The model under review builds one solid part; all positions refer to its coordinate system, in mm. A direction names the side the tool comes from. Give positions to 0.01 mm unless a question says otherwise; leave off trailing zeros. Order: outer loops, then holes, each group sorted by start corner. A loop starts at its lowest first (then second) coordinate and runs counter-clockwise, first axis right, second up.
```python
from build123d import *

# Parameters (mm, degrees)
SKETCH1_W           = 10
SKETCH1_H           = 4
BOSS_EXTRUDE1_DEPTH = 1
SKETCH1_3_W         = 38
SKETCH1_3_H         = 1
BOSS_EXTRUDE2_DEPTH = 4
BOSS_EXTRUDE3_DEPTH = 23
SKETCH2_W           = 5
SKETCH2_H           = 3
BOSS_EXTRUDE4_DEPTH = 3
CUT_EXTRUDE1_DEPTH  = 56.873182297
BOSS_EXTRUDE5_DEPTH = 7
BOSS_EXTRUDE8_DEPTH = 23
SKETCH6_W           = 5
SKETCH6_H           = 3
BOSS_EXTRUDE9_DEPTH = 3
CUT_EXTRUDE3_DEPTH  = 56.873182297


with BuildPart() as part:
    # Sketch1 → Boss-Extrude1 (new body)
    with BuildSketch(Plane(origin=(0, 0, 0), x_dir=(1, 0, 0), z_dir=(0, 1, 0))):
        with BuildLine():
            Line((8.75, 22.5), (8.75, 12))
            ThreePointArc((8.75, 12), (8.530330086, 11.469669914), (8, 11.25))
            Line((8, 11.25), (0.75, 11.25))
            ThreePointArc((0.75, 11.25), (0.219669914, 11.469669914), (0, 12))
            Line((0, 12), (0, 1))
            ThreePointArc((0, 1), (0.292893219, 0.292893219), (1, 0))
            Line((1, 0), (43, 0))
            ThreePointArc((43, 0), (43.707106781, 0.292893219), (44, 1))
            Line((44, 1), (44, 33.5))
            ThreePointArc((44, 33.5), (43.707106781, 34.207106781), (43, 34.5))
            Line((43, 34.5), (1, 34.5))
            ThreePointArc((1, 34.5), (0.292893219, 34.207106781), (0, 33.5))
            Line((0, 33.5), (0, 22.5))
            ThreePointArc((0, 22.5), (0.219669914, 23.030330086), (0.75, 23.25))
            Line((0.75, 23.25), (8, 23.25))
            ThreePointArc((8, 23.25), (8.530330086, 23.030330086), (8.75, 22.5))
        make_face()
        with Locations((33.2, 26.7)):
            Rectangle(SKETCH1_W, SKETCH1_H, mode=Mode.SUBTRACT)
    extrude(amount=BOSS_EXTRUDE1_DEPTH)

    # Sketch1<3> → Boss-Extrude2 (add)
    # profile 1 of 12: a face of its own
    with BuildSketch(Plane(origin=(0, 0, 0), x_dir=(1, 0, 0), z_dir=(0, 1, 0))):
        with BuildLine():
            ThreePointArc((43.5, 35.5), (44.560660172, 35.060660172), (45, 34))
            Line((45, 34), (45, 0.5))
            ThreePointArc((45, 0.5), (44.560660172, -0.560660172), (43.5, -1))
            Line((43.5, -1), (0.5, -1))
            ThreePointArc((0.5, -1), (-0.560660172, -0.560660172), (-1, 0.5))
            Line((-1, 0.5), (-1, 34))
            ThreePointArc((-1, 34), (-0.560660172, 35.060660172), (0.5, 35.5))
            Line((0.5, 35.5), (43.5, 35.5))
        make_face()
        with BuildLine():
            ThreePointArc((1, 34.5), (0.292893219, 34.207106781), (0, 33.5))
            Line((0, 33.5), (0, 24.75))
            Line((0, 24.75), (0, 22.5))
            Line((0, 22.5), (0, 12))
            Line((0, 12), (0, 9.75))
            Line((0, 9.75), (0, 1))
            ThreePointArc((0, 1), (0.292893219, 0.292893219), (1, 0))
            Line((1, 0), (43, 0))
            ThreePointArc((43, 0), (43.707106781, 0.292893219), (44, 1))
            Line((44, 1), (44, 33.5))
            ThreePointArc((44, 33.5), (43.707106781, 34.207106781), (43, 34.5))
            Line((43, 34.5), (1, 34.5))
        make_face(mode=Mode.SUBTRACT)
    # profile 2 of 12: a face of its own
    with BuildSketch(Plane(origin=(0, 0, 0), x_dir=(1, 0, 0), z_dir=(0, 1, 0))):
        with BuildLine():
            Line((3, 0), (1, 0))
            ThreePointArc((1, 0), (0.292893219, 0.292893219), (0, 1))
            Line((0, 1), (0, 3))
            Line((0, 3), (-1, 3))
            Line((-1, 3), (-1, 0.5))
            ThreePointArc((-1, 0.5), (-0.560660172, -0.560660172), (0.5, -1))
            Line((0.5, -1), (3, -1))
            Line((3, -1), (3, 0))
        make_face()
    # profile 3 of 12: a face of its own
    with BuildSketch(Plane(origin=(0, 0, 0), x_dir=(1, 0, 0), z_dir=(0, 1, 0))):
        with Locations((22, -0.5)):
            Rectangle(SKETCH1_3_W, SKETCH1_3_H)
    # profile 4 of 12: a face of its own
    with BuildSketch(Plane(origin=(0, 0, 0), x_dir=(1, 0, 0), z_dir=(0, 1, 0))):
        with BuildLine():
            Line((43, 0), (41, 0))
            Line((41, 0), (41, -1))
            Line((41, -1), (43.5, -1))
            ThreePointArc((43.5, -1), (44.560660172, -0.560660172), (45, 0.5))
            Line((45, 0.5), (45, 3))
            Line((45, 3), (44, 3))
            Line((44, 3), (44, 1))
            ThreePointArc((44, 1), (43.707106781, 0.292893219), (43, 0))
        make_face()
    # profile 5 of 12: a face of its own
    with BuildSketch(Plane(origin=(0, 0, 0), x_dir=(1, 0, 0), z_dir=(0, 1, 0))):
        with BuildLine():
            Line((44, 14.75), (44, 3))
            Line((44, 3), (45, 3))
            Line((45, 3), (45, 14.958712153))
            ThreePointArc((45, 14.958712153), (44.510774109, 14.802734218), (44, 14.75))
        make_face()
    # profile 6 of 12: a face of its own
    with BuildSketch(Plane(origin=(0, 0, 0), x_dir=(1, 0, 0), z_dir=(0, 1, 0))):
        with BuildLine():
            Line((44, 31.5), (44, 19.75))
            ThreePointArc((44, 19.75), (44.510774109, 19.697265782), (45, 19.541287847))
            Line((45, 19.541287847), (45, 31.5))
            Line((45, 31.5), (44, 31.5))
        make_face()
    # profile 7 of 12: a face of its own
    with BuildSketch(Plane(origin=(0, 0, 0), x_dir=(1, 0, 0), z_dir=(0, 1, 0))):
        with BuildLine():
            Line((44, 19.75), (44, 14.75))
            ThreePointArc((44, 14.75), (44.510774109, 14.802734218), (45, 14.958712153))
            Line((45, 14.958712153), (45, 19.541287847))
            ThreePointArc((45, 19.541287847), (44.510774109, 19.697265782), (44, 19.75))
        make_face()
    # profile 8 of 12: a face of its own
    with BuildSketch(Plane(origin=(0, 0, 0), x_dir=(1, 0, 0), z_dir=(0, 1, 0))):
        with BuildLine():
            Line((44, 33.5), (44, 31.5))
            Line((44, 31.5), (45, 31.5))
            Line((45, 31.5), (45, 34))
            ThreePointArc((45, 34), (44.560660172, 35.060660172), (43.5, 35.5))
            Line((43.5, 35.5), (41, 35.5))
            Line((41, 35.5), (41, 34.5))
            Line((41, 34.5), (43, 34.5))
            ThreePointArc((43, 34.5), (43.707106781, 34.207106781), (44, 33.5))
        make_face()
    # profile 9 of 12: a face of its own
    with BuildSketch(Plane(origin=(0, 0, 0), x_dir=(1, 0, 0), z_dir=(0, 1, 0))):
        with Locations((22, 35)):
            Rectangle(SKETCH1_3_W, SKETCH1_3_H)
    # profile 10 of 12: a face of its own
    with BuildSketch(Plane(origin=(0, 0, 0), x_dir=(1, 0, 0), z_dir=(0, 1, 0))):
        with BuildLine():
            Line((-1, 34), (-1, 31.5))
            Line((-1, 31.5), (0, 31.5))
            Line((0, 31.5), (0, 33.5))
            ThreePointArc((0, 33.5), (0.292893219, 34.207106781), (1, 34.5))
            Line((1, 34.5), (3, 34.5))
            Line((3, 34.5), (3, 35.5))
            Line((3, 35.5), (0.5, 35.5))
            ThreePointArc((0.5, 35.5), (-0.560660172, 35.060660172), (-1, 34))
        make_face()
    # profile 11 of 12: a face of its own
    with BuildSketch(Plane(origin=(0, 0, 0), x_dir=(1, 0, 0), z_dir=(0, 1, 0))):
        with BuildLine():
            Line((-1, 3), (0, 3))
            Line((0, 3), (0, 9.75))
            Line((0, 9.75), (0, 12))
            Line((0, 12), (0, 14.75))
            ThreePointArc((0, 14.75), (-0.510774109, 14.802734218), (-1, 14.958712153))
            Line((-1, 14.958712153), (-1, 3))
        make_face()
    # profile 12 of 12: a face of its own
    with BuildSketch(Plane(origin=(0, 0, 0), x_dir=(1, 0, 0), z_dir=(0, 1, 0))):
        with BuildLine():
            Line((-1, 31.5), (-1, 19.541287847))
            ThreePointArc((-1, 19.541287847), (-0.510774109, 19.697265782), (0, 19.75))
            Line((0, 19.75), (0, 22.5))
            Line((0, 22.5), (0, 24.75))
            Line((0, 24.75), (0, 31.5))
            Line((0, 31.5), (-1, 31.5))
        make_face()
    extrude(amount=BOSS_EXTRUDE2_DEPTH)

    # Sketch1<4> → Boss-Extrude3 (add)
    with BuildSketch(Plane(origin=(0, 0, 0), x_dir=(1, 0, 0), z_dir=(0, 1, 0))):
        with BuildLine():
            Line((45, 19.541287847), (45, 14.958712153))
            ThreePointArc((45, 14.958712153), (46.5, 17.25), (45, 19.541287847))
        make_face()
        with BuildLine():
            Line((44, 19.75), (44, 14.75))
            ThreePointArc((44, 14.75), (44.510774109, 14.802734218), (45, 14.958712153))
            Line((45, 14.958712153), (45, 19.541287847))
            ThreePointArc((45, 19.541287847), (44.510774109, 19.697265782), (44, 19.75))
        make_face()
    extrude(amount=BOSS_EXTRUDE3_DEPTH)

    # Sketch2 → Boss-Extrude4 (add)
    with BuildSketch(Plane.ZY.offset(-44)):
        with Locations((-17.25, 21.5)):
            Rectangle(SKETCH2_W, SKETCH2_H)
    extrude(amount=BOSS_EXTRUDE4_DEPTH)

    # Sketch3 → Cut-Extrude1 (cut, through all)
    with BuildSketch(Plane.XY.offset(-14.75)):
        Polygon((41, 20), (44, 23), (41, 23), align=None)
    extrude(amount=-CUT_EXTRUDE1_DEPTH, mode=Mode.SUBTRACT)

    # Sketch1<6> → Boss-Extrude5 (add)
    with BuildSketch(Plane(origin=(0, 0, 0), x_dir=(1, 0, 0), z_dir=(0, 1, 0))):
        with BuildLine():
            Line((-1, 34), (-1, 31.5))
            Line((-1, 31.5), (0, 31.5))
            Line((0, 31.5), (0, 33.5))
            ThreePointArc((0, 33.5), (0.292893219, 34.207106781), (1, 34.5))
            Line((1, 34.5), (3, 34.5))
            Line((3, 34.5), (3, 35.5))
            Line((3, 35.5), (0.5, 35.5))
            ThreePointArc((0.5, 35.5), (-0.560660172, 35.060660172), (-1, 34))
        make_face()
        with BuildLine():
            Line((3, 0), (1, 0))
            ThreePointArc((1, 0), (0.292893219, 0.292893219), (0, 1))
            Line((0, 1), (0, 3))
            Line((0, 3), (-1, 3))
            Line((-1, 3), (-1, 0.5))
            ThreePointArc((-1, 0.5), (-0.560660172, -0.560660172), (0.5, -1))
            Line((0.5, -1), (3, -1))
            Line((3, -1), (3, 0))
        make_face()
        with BuildLine():
            Line((43, 0), (41, 0))
            Line((41, 0), (41, -1))
            Line((41, -1), (43.5, -1))
            ThreePointArc((43.5, -1), (44.560660172, -0.560660172), (45, 0.5))
            Line((45, 0.5), (45, 3))
            Line((45, 3), (44, 3))
            Line((44, 3), (44, 1))
            ThreePointArc((44, 1), (43.707106781, 0.292893219), (43, 0))
        make_face()
        with BuildLine():
            Line((44, 33.5), (44, 31.5))
            Line((44, 31.5), (45, 31.5))
            Line((45, 31.5), (45, 34))
            ThreePointArc((45, 34), (44.560660172, 35.060660172), (43.5, 35.5))
            Line((43.5, 35.5), (41, 35.5))
            Line((41, 35.5), (41, 34.5))
            Line((41, 34.5), (43, 34.5))
            ThreePointArc((43, 34.5), (43.707106781, 34.207106781), (44, 33.5))
        make_face()
    extrude(amount=BOSS_EXTRUDE5_DEPTH)

    # Sketch1<9> → Boss-Extrude8 (add)
    with BuildSketch(Plane(origin=(0, 0, 0), x_dir=(1, 0, 0), z_dir=(0, 1, 0))):
        with BuildLine():
            ThreePointArc((-1, 19.541287847), (-2.5, 17.25), (-1, 14.958712153))
            Line((-1, 14.958712153), (-1, 19.541287847))
        make_face()
        with BuildLine():
            Line((-1, 19.541287847), (-1, 14.958712153))
            ThreePointArc((-1, 14.958712153), (-0.510774109, 14.802734218), (0, 14.75))
            Line((0, 14.75), (0, 19.75))
            ThreePointArc((0, 19.75), (-0.510774109, 19.697265782), (-1, 19.541287847))
        make_face()
    extrude(amount=BOSS_EXTRUDE8_DEPTH)

    # Sketch6 → Boss-Extrude9 (add)
    with BuildSketch(Plane(origin=(0, 0, 0), x_dir=(0, 0, -1), z_dir=(1, 0, 0))):
        with Locations((17.25, 21.5)):
            Rectangle(SKETCH6_W, SKETCH6_H)
    extrude(amount=BOSS_EXTRUDE9_DEPTH)

    # Sketch7 → Cut-Extrude3 (cut, through all)
    with BuildSketch(Plane.XY.offset(-14.75)):
        Polygon((3, 23), (3, 20), (0, 23), align=None)
    extrude(amount=-CUT_EXTRUDE3_DEPTH, mode=Mode.SUBTRACT)


solid = part.part
```
1. Insertion check: pin 1 (1.5 mm diameter, centred on x = 1.5, y = 21, fed in from +Z); pin 2 (10 mm diameter, centred on x = 8, y = 4.5, fed in from -Z); pin 3 (7.5 mm diameter, centred on y = 4, z = -29, fed in from -X); pin 4 (0.9 mm diameter, centred on x = 2, y = 21.5, fed in from -Z). Each pin has a flat end and moves straight along its axis. Give the tip position at first contact, or say it passes through.
2. For faces 1 (the cylindrical face through (43.699, 3.958, -0.285)), 2 (the flat face through (0, 7, 0)), 3 (the flat face through (43, 20, -17)), 4 (the flat face through (41, 5, -35)), 5 (the flat face through (-0.5, 5.5, -3)), list the 3-axis set-ups (+Z, -Z, +X, -X, +Y, -Y) from which the entire face can be reached by the end or side of a thin tool; tool diameter is ignored.
3. Take a section at B-B (y = 3.25). Write out the cut boundary in (x, z), and give its area (3 significant figures).
4. Take a section at A-A (x = 29.5). Write out the cut boundary in (y, z), and give its area (3 significant figures).
5. Take a section at D-D (y = 16.75). Write out the cut boundary in (x, z).
6. To check wall thickness, follow line 1 (Y direction, x = 31, z = -23); line 2 (X direction, y = 16.5, z = -18.5). State the ranges of each line that lie inside material, in increasing order.
7. Take a section at C-C (z = -24). Write out the cut boundary in (x, y), and give its area (3 significant figures).
8. Draft analysis for pull direction X (two halves, no side actions). For faces 6 (the flat face through (44.5, 4, -25.6)), 7 (the cylindrical face through (44.57, 3.45, 0.55)), 8 (the flat face through (3, 5.5, 0.5)), state which applies: pulls with the +X half, pulls with the -X half, needs draft (parallel to the pull), parting line crosses it, or undercut.
Answer:
1. pin 1: stops at z = -14.75
1. pin 2: stops at z = -35.5
1. pin 3: stops at x = -1
1. pin 4: stops at z = -19.75
2. face 1: +Y
2. face 2: +Z, +X, -X, +Y
2. face 3: +Z, -Z
2. face 4: +Z, -Z, +Y
2. face 5: +X, -X, +Y
3. outline: (-1, -34) arc R1.5 ccw to (0.5, -35.5) - (43.5, -35.5) arc R1.5 ccw to (45, -34) - (45, -19.54) arc R2.5 ccw to (45, -14.96) - (45, -0.5) arc R1.5 ccw to (43.5, 1) - (0.5, 1) arc R1.5 ccw to (-1, -0.5) - (-1, -14.96) arc R2.5 ccw to (-1, -19.54) - close; hole (0, -33.5) arc R1 ccw to (1, -34.5) - (43, -34.5) arc R1 ccw to (44, -33.5) - (44, -1) arc R1 ccw to (43, 0) - (1, 0) arc R1 ccw to (0, -1) - close
3. area: 170 mm2
4. outline: (0, -35.5) - (4, -35.5) - (4, -34.5) - (1, -34.5) - (1, -28.7) - (0, -28.7) - close; (0, -24.7) - (1, -24.7) - (1, 0) - (4, 0) - (4, 1) - (0, 1) - close
4. area: 38.5 mm2
5. outline: (0, -19.75) - (0, -14.75) arc R2.5 ccw to start; (44, -19.75) arc R2.5 ccw to (44, -14.75) - close
6. line 1: y = 0 to 1
6. line 2: x = -2.17 to 0, 44 to 46.17
7. outline: (-1, 0) - (45, 0) - (45, 4) - (44, 4) - (44, 1) - (0, 1) - (0, 4) - (-1, 4) - close
7. area: 52.0 mm2
8. face 6: needs draft
8. face 7: pulls with the +X half
8. face 8: undercut
